The figure shows three views and two pictorial views of one solid part (mm, origin at its lowest corner). Answer the questions. A direction names the side the tool comes from. Coordinates: 2 decimals unless noted, no trailing zeros. Order: outer loops, then holes, each group sorted by start corner. A loop starts at its lowest first (then second) coordinate and runs counter-clockwise, first axis right, second up. Notation, with made-up numbers: M 5,-21.5 L 39,-21.5 A33 cw 39,14.5 Z; hole C 39.5,-4 d9. An arc over 180 degrees is marked long. Write item = value, one per line. Start each with the question number.
Q1. Find section D-D on z = 3.95. Give the vertices of the cut face in (x, y).
Q2. Find section B-B on x = 6.5. Give the vertices of the cut face in (y, z).
Q3. Find section C-C on y = 12.5. Give the vertices of the cut face in (x, z), and give its area (3 significant figures).
Q4. A tool of negligible diameter and unlimited length cuts with its end or side. For the marked faces 4, 5 and 6, from which of +Z, -Z, +X, -X, +Y, -Y can it reach the whole face along a straight path? Write none if from no direction.
Q5. Determine the mould class of the marked faces 1, 2 and 3 for opening direction X: released by +X, released by -X, zero draft, split by the parting line, or undercut.
Q6. Each of these flat-tipped pins is pushed along its axis until it touches: P1, Ø1, axis at x = 5.5, z = 1, coming from the +Y side; P2, Ø0.8, axis at x = 15, z = 2.5, coming from the +Y side; P3, Ø3, axis at x = 9.5, y = 9, coming from the -Z side. Where does it stop, or does it pass through?
Q7. Find section A-A on z = 2.05. Give the vertices of the cut face in (x, y).
Q8. Straight lines are drawn through the part: line 1 along X through (y, z) = (8.75, 3.1); line 2 along Z through (x, y) = (10, 6); line 3 along Z through (x, y) = (14.5, 9.5). For each, find the intervals that lie inside material, in ascending order.
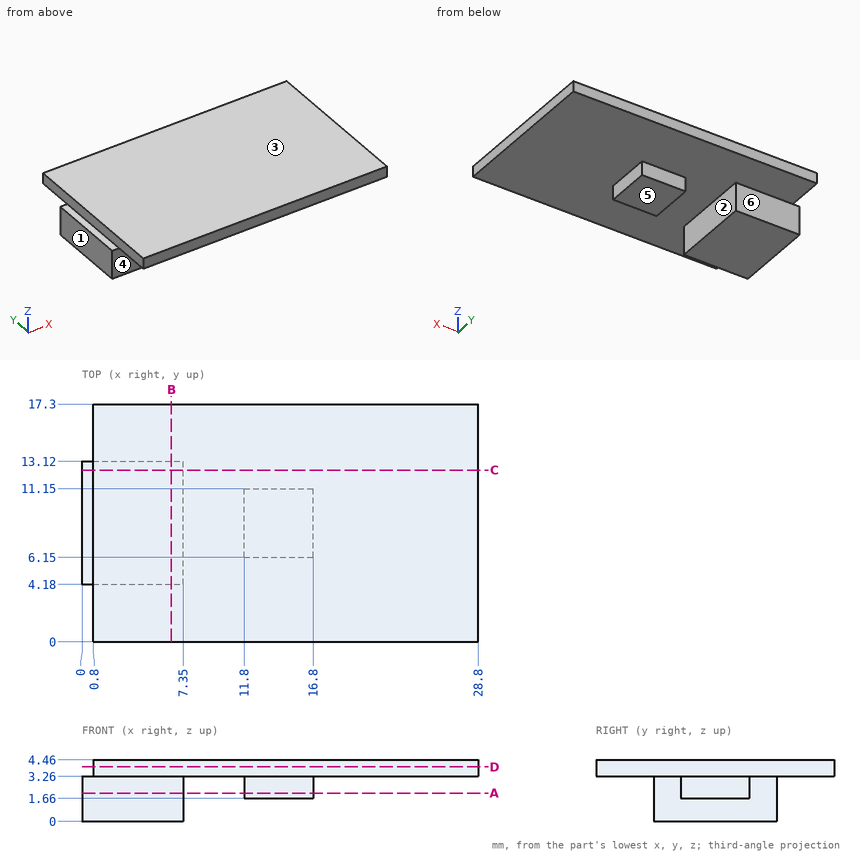
Findings below:
q1.outline = M 0.8,0 L 28.8,0 L 28.8,17.3 L 0.8,17.3 Z
q2.outline = M 0,3.26 L 4.18,3.26 L 4.18,0 L 13.12,0 L 13.12,3.26 L 17.3,3.26 L 17.3,4.46 L 0,4.46 Z
q3.outline = M 0,0 L 7.35,0 L 7.35,3.26 L 28.8,3.26 L 28.8,4.46 L 0.8,4.46 L 0.8,3.26 L 0,3.26 Z
q3.area = 57.6 mm^2
q4.face_4 = -Z, +X, -X, -Y
q4.face_5 = -Z, +X, +Y, -Y
q4.face_6 = -Z, +X, -X, +Y
q5.face_1 = released by -X
q5.face_2 = undercut
q5.face_3 = zero draft
q6.P1 = 13.12
q6.P2 = 11.15
q6.P3 = 3.26
q7.outline = M 0,4.18 L 7.35,4.18 L 7.35,13.12 L 0,13.12 Z; M 11.8,6.15 L 16.8,6.15 L 16.8,11.15 L 11.8,11.15 Z
q8.line_1 = 0 to 7.35, 11.8 to 16.8
q8.line_2 = 3.26 to 4.46
q8.line_3 = 1.66 to 4.46
